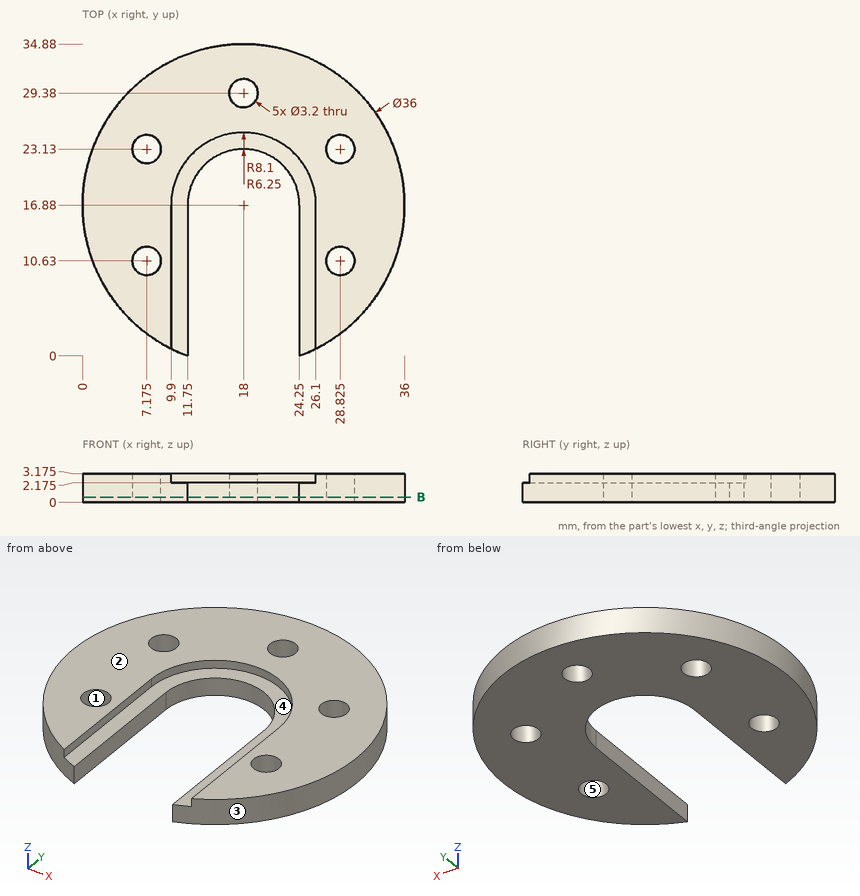
Study the drawing (mm; zero at the part's minimum x, y, z) and answer. A direction names the side the tool comes from. Coordinates: 2 decimals unless noted, no trailing zeros. Answer in a Markdown table with one row per item. Add a question column.
1. Consider line 1 (X direction, y = 17, z = 1.1); line 2 (Y direction, x = 6.5, z = 2.25); line 3 (Y direction, x = 7.5, z = 0.7) (1 decimal). Determine where each line is inside the solid, lowest interval first. Write a range as [from, to].
2. The part is cut by section B-B, the plane z = 0.6. Count the separate pieces of the cut face and the enclosed holes in it, then the cut area to 3 significant figures.
3. Flat-ended cylindrical pins translate along their axes: P1, Ø6, axis at x = 20.5, y = 10.5, coming from the +Z side; P2, Ø1.1, axis at y = 12, z = 3, coming from the -X side; P3, Ø0.5, axis at y = 7, z = 3, coming from the +X side; P4, Ø1.1, axis at y = 5.5, z = 1, coming from the +X side. Find the tip coordinate at first contact, or state that the pin passes through.
4. For the marked faces 4 and 5, determine the directions among +Z, -Z, +X, -X, +Y, -Y from which every point of the face is accessible in a straight line to the end or side of a thin tool.
5. Determine the mould class of the marked faces 1, 2 and 3 for opening direction X: +X half, -X half, draft (parallel to the pull), parting line (faces both ways), or undercut.
Answer below:
| question | item | result |
|---|---|---|
| 1 | line 1 | [0, 11.75], [24.25, 36] |
| 1 | line 2 | [3.03, 9.18], [12.08, 21.68], [24.58, 30.73] |
| 1 | line 3 | [2.3, 9.1], [12.2, 21.6], [24.7, 31.5] |
| 2 | separate pieces | 1 |
| 2 | enclosed holes | 5 |
| 2 | area | 696 mm2 |
| 3 | P1 | through |
| 3 | P2 | x = 0.53 |
| 3 | P3 | x = 33.21 |
| 3 | P4 | x = 32.38 |
| 4 | face 4 | +Z, -Y |
| 4 | face 5 | +Z, -Z |
| 5 | face 1 | undercut |
| 5 | face 2 | draft |
| 5 | face 3 | parting line |
